Can you work these out from the model? Positions are in its coordinate system, mm. Face numbers are marked on the shaded views. A direction names the side the tool comes from. Give positions to 0.01 mm unless a question says otherwise; leave off trailing zeros. Loops run counter-clockwise (first coordinate to the right, second up) from the corner with the lowest first, then second, coordinate; pieces in that order, holes last. Notation, with made-up numbers: (20.5, -19.5) - (24.5, -19.5) arc R18 cw to (24.5, -0.5) - close; hole circle Ø9 at (55.25, 35.25). An arc over 180 degrees is marked (long way). Write item = value, one per line.
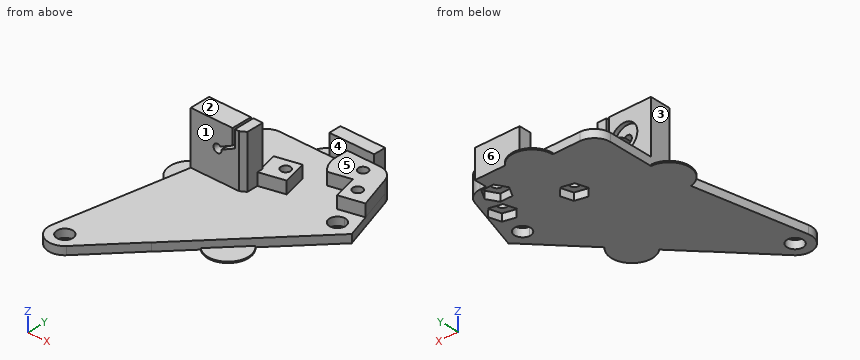
from build123d import *

# Parameters (mm, degrees)
SKETCH2_R                = 3.81
BOSS_EXTRUDE1_DEPTH      = 2.54
SKETCH5_W                = 16.764
SKETCH5_H                = 6.35
BOSS_EXTRUDE2_DEPTH      = 16.51
SKETCH6_R                = 4.1275
CUT_EXTRUDE2_DEPTH       = 1.27
SKETCH7_R                = 1.27
CUT_EXTRUDE3_DEPTH       = 65.77
CUT_EXTRUDE4_DEPTH       = 2.286
BOSS_EXTRUDE3_DEPTH      = 3.81
F_4_CLEARANCE_HOLE1_D    = 2.9464
SKETCH14_W               = 13.97
SKETCH14_H               = 3.81
BOSS_EXTRUDE6_DEPTH      = 6.35
BOSS_EXTRUDE6_DEPTH_BACK = 2.54
FILLET1_R                = 5.08
CUT_EXTRUDE5_DEPTH       = 17.51
CUT_EXTRUDE5_DEPTH_BACK  = 3.54
SKETCH19_R               = 2.4892
BOSS_EXTRUDE8_DEPTH      = 2.54
CUT_EXTRUDE8_DEPTH       = 2.54
CUT_EXTRUDE9_DEPTH       = 53.355501773
SKETCH13_R               = 6.35
PRINT_TABS_DEPTH         = 0.4


with BuildPart() as part:
    # Sketch2 → Boss-Extrude1 (new body)
    with BuildSketch(Plane.XY):
        with BuildLine():
            Line((-17.068825413, -8.459178389), (-41.402, 40.64))
            Line((-41.402, 40.64), (-41.402, 66.04))
            Line((-41.402, 66.04), (-1.524, 66.04))
            Line((-1.524, 66.04), (18.109053667, 5.913093546))
            ThreePointArc((18.109053667, 5.913093546), (7.204933647, -17.634949139), (-17.068825413, -8.459178389))
        make_face()
        Circle(SKETCH2_R, mode=Mode.SUBTRACT)
    extrude(amount=BOSS_EXTRUDE1_DEPTH)

    # Sketch5 → Boss-Extrude2 (add)
    with BuildSketch(Plane.XY.offset(2.54)):
        with Locations((-33.02, 43.815)):
            Rectangle(SKETCH5_W, SKETCH5_H)
    extrude(amount=BOSS_EXTRUDE2_DEPTH)

    # Sketch6 → Cut-Extrude2 (cut)
    with BuildSketch(Plane(origin=(0, 46.99, 0), x_dir=(1, 0, 0), z_dir=(0, 1, 0))):
        with Locations((-33.02, -11.43)):
            Circle(SKETCH6_R)
    extrude(amount=-CUT_EXTRUDE2_DEPTH, mode=Mode.SUBTRACT)

    # Sketch7 → Cut-Extrude3 (cut, through all)
    with BuildSketch(Plane(origin=(0, 45.72, 0), x_dir=(1, 0, 0), z_dir=(0, 1, 0))):
        with Locations((-33.02, -11.43)):
            Circle(SKETCH7_R)
    extrude(amount=-CUT_EXTRUDE3_DEPTH, mode=Mode.SUBTRACT)

    # Sketch9 → Cut-Extrude4 (cut)
    with BuildSketch(Plane(origin=(0, 0, 0), x_dir=(-1, 0, 0), z_dir=(0, 0, -1))):
        Polygon((3.171122265, 62.23), (5.077532854, 58.928), (8.890354032, 58.928), (10.796764621, 62.23), (8.890354032, 65.532), (5.077532854, 65.532), align=None)
        Polygon((24.379877895, 49.663956202), (23.308143816, 53.323053276), (19.603405755, 54.224452874), (16.970401774, 51.466755398), (18.042135853, 47.807658324), (21.746873914, 46.906258726), align=None)
        Polygon((5.918476139, 54.15579827), (4.846742059, 57.814895344), (1.142003999, 58.716294942), (-1.490999983, 55.958597466), (-0.419265903, 52.299500392), (3.285472157, 51.398100794), align=None)
    extrude(amount=-CUT_EXTRUDE4_DEPTH, mode=Mode.SUBTRACT)

    # Sketch8 → Boss-Extrude3 (add)
    with BuildSketch(Plane.XY.offset(2.54)):
        with BuildLine():
            Line((-15.367, 66.04), (-6.983943443, 66.04))
            Line((-6.983943443, 66.04), (-1.524, 66.04))
            Line((-1.524, 66.04), (3.09175139, 51.904101595))
            Line((3.09175139, 51.904101595), (-4.240438106, 50.120107003))
            Line((-4.240438106, 50.120107003), (-6.088713216, 57.716488409))
            Line((-6.088713216, 57.716488409), (-12.708473154, 56.10583501))
            ThreePointArc((-12.708473154, 56.10583501), (-14.673699407, 58.891843255), (-15.367, 62.23))
            Line((-15.367, 62.23), (-15.367, 66.04))
        make_face()
        Polygon((-17.142042414, 46.981018422), (-18.990317524, 54.577399829), (-26.415687706, 52.770733449), (-24.567412596, 45.174352043), align=None)
    extrude(amount=BOSS_EXTRUDE3_DEPTH)

    # #4 Clearance Hole1 (through all)
    with Locations(Plane.XY.offset(6.35)):
        with Locations((-6.983943443, 62.23), (-20.675139834, 50.5653558), (-2.213738078, 55.057197868)):
            Hole(F_4_CLEARANCE_HOLE1_D / 2)

    # Sketch14 → Boss-Extrude6 (add, two sides)
    with BuildSketch(Plane.XY.offset(2.54)) as boss_extrude6_sk:
        with Locations((-13.968943443, 67.945)):
            Rectangle(SKETCH14_W, SKETCH14_H)
    extrude(amount=BOSS_EXTRUDE6_DEPTH)
    extrude(boss_extrude6_sk.sketch, amount=-BOSS_EXTRUDE6_DEPTH_BACK)

    # Fillet1
    fillet1_edges = [part.edges().sort_by_distance(p)[0] for p in [
        (-1.524, 66.04, 3.175),
        (-41.402, 66.04, 1.27),
    ]]
    fillet(fillet1_edges, radius=FILLET1_R)

    # Sketch15 → Cut-Extrude5 (cut, two sides)
    with BuildSketch(Plane.XY.offset(2.54)) as cut_extrude5_sk:
        with BuildLine():
            ThreePointArc((-0.315167053, 48.411374113), (-18.310138041, 44.816284079), (-33.674369734, 34.782140486))
            ThreePointArc((-33.674369734, 34.782140486), (-33.731327517, 31.262340905), (-30.211527936, 31.205383122))
            ThreePointArc((-30.211527936, 31.205383122), (-16.427248714, 40.207684038), (-0.28275743, 43.433079608))
            ThreePointArc((-0.28275743, 43.433079608), (2.190185011, 45.938431672), (-0.315167053, 48.411374113))
        make_face()
    extrude(amount=CUT_EXTRUDE5_DEPTH, mode=Mode.SUBTRACT)
    extrude(cut_extrude5_sk.sketch, amount=-CUT_EXTRUDE5_DEPTH_BACK, mode=Mode.SUBTRACT)

    # Sketch19 → Boss-Extrude8 (add, through all)
    with BuildSketch(Plane.XY.offset(2.54)):
        with BuildLine():
            Line((5.466200245, 44.632269783), (-40.158007355, -3.769954845))
            ThreePointArc((-40.158007355, -3.769954845), (-46.15516131, -4.814733016), (-48.848797168, 0.64436424))
            Line((-48.848797168, 0.64436424), (-41.402, 40.64))
            Line((-41.402, 40.64), (3.09175139, 51.904101595))
            Line((3.09175139, 51.904101595), (5.466200245, 44.632269783))
        make_face()
        with Locations((-0.298962241, 45.92222686)):
            Circle(SKETCH19_R, mode=Mode.SUBTRACT)
        with Locations((-43.854625645, -0.285501773)):
            Circle(SKETCH19_R, mode=Mode.SUBTRACT)
    extrude(amount=-BOSS_EXTRUDE8_DEPTH)

    # Sketch20 → Cut-Extrude8 (cut)
    with BuildSketch(Plane.XY.offset(2.54)):
        Polygon((-40.158007355, -3.769954845), (10.729493517, 49.863783044), (48.07174347, 14.433588323), (-7.673080914, -44.319607422), align=None)
    extrude(amount=-CUT_EXTRUDE8_DEPTH, mode=Mode.SUBTRACT)

    # Sketch21 → Cut-Extrude9 (cut, through all)
    with BuildSketch(Plane(origin=(0, 46.99, 0), x_dir=(1, 0, 0), z_dir=(0, 1, 0))):
        Polygon((-27.559, -19.05), (-27.559, -13.73452905), (-32.84961162, -11.08922324), (-33.19038838, -11.77077676), (-28.321, -14.20547095), (-28.321, -19.05), align=None)
    extrude(amount=-CUT_EXTRUDE9_DEPTH, mode=Mode.SUBTRACT)

    # Sketch13 → Print Tabs (add)
    with BuildSketch(Plane(origin=(0, 0, 0), x_dir=(-1, 0, 0), z_dir=(0, 0, -1))):
        with Locations((14.284313144, 23.500060577)):
            Circle(SKETCH13_R)
        with Locations((21.463, 66.04)):
            Circle(SKETCH13_R)
        with Locations((41.402, 40.64)):
            Circle(SKETCH13_R)
    extrude(amount=-PRINT_TABS_DEPTH)


solid = part.part
Q1. We'd pull the mould along Y, two halves only. Please class the marked faces 4, 5 and 6: released by +Y, released by -Y, zero draft, split by the parting line, or undercut.
Output:
face_4 = undercut
face_5 = zero draft
face_6 = released by +Y
Q2. Imagine slicing it at B-B, the plane z = 18. Write out the boundary of the cut face in (x, y), then the cut area to 3 significant figures.
Output:
outline = (-41.4, 40.64) - (-28.32, 40.64) - (-28.32, 46.99) - (-41.4, 46.99) - close; (-27.56, 40.64) - (-26.31, 40.64) arc R48.41 cw to (-24.64, 41.67) - (-24.64, 46.99) - (-27.56, 46.99) - close
area = 101 mm2
Q3. Imagine slicing it at D-D, the plane x = -2. Write out the boundary of the cut face in (y, z), then the cut area to 3 significant figures.
Output:
outline = (36.45, 0) - (44.1, 0) - (44.1, 2.54) - (36.45, 2.54) - close; (47.74, 0) - (51.71, 0) - (51.71, 2.29) - (53.6, 2.29) - (53.6, 6.35) - (50.67, 6.35) - (50.67, 2.54) - (47.74, 2.54) - close; (56.51, 2.29) - (58.51, 2.29) - (58.51, 0) - (64.9, 0) - (64.9, 6.35) - (56.51, 6.35) - close
area = 89.9 mm2
Q4. For pin 1 (4 mm diameter, centred on y = 63, z = 4, fed in from -X); pin 2 (7.5 mm diameter, centred on x = -33.02, z = 11.43, fed in from +Y); pin 3 (1.9 mm diameter, centred on x = -14.5, z = 6.5, fed in from -Y); pin 4 (6 mm diameter, centred on y = 37, z = 15.5, fed in from +X), each with a flat end and sliding along its axis, tell me the tip position at first contact or that it passes through.
Output:
pin_1 = -41.36
pin_2 = 45.72
pin_3 = 57.03
pin_4 = through
Q5. Imagine slicing it at C-C, the plane z = 4.75. Write out the boundary of the cut face in (x, y), then the cut area to 3 significant figures.
Output:
outline = (-41.4, 40.64) - (-26.31, 40.64) arc R48.41 cw to (-24.64, 41.67) - (-24.64, 45.46) - (-24.57, 45.17) - (-17.14, 46.98) - (-18.99, 54.58) - (-26.42, 52.77) - (-25.01, 46.99) - (-41.4, 46.99) - close; (-20.95, 66.04) - (-15.37, 66.04) - (-15.37, 62.23) arc R8.38 ccw to (-12.71, 56.11) - (-6.09, 57.72) - (-4.24, 50.12) - (3.09, 51.9) - (-0.38, 62.54) arc R5.08 ccw to (-5.21, 66.04) - (-6.98, 66.04) - (-6.98, 69.85) - (-20.95, 69.85) - close; hole circle Ø2.95 at (-20.68, 50.57); hole circle Ø2.95 at (-6.98, 62.23); hole circle Ø2.95 at (-2.21, 55.06)
area = 377 mm2
Q6. I need wall thicknesses on L1, parallel to X at y = 44.3, z = 11.43; L2, parallel to Z at x = -33.02, y = 43.3; L3, parallel to Z at x = -33.5, y = 60. Which ranges of each line are inside material? Lowest first, please.
Output:
L1 = -41.4 to -34.29, -31.75 to -24.64
L2 = 0 to 10.16, 12.7 to 19.05
L3 = 0 to 2.54
Q7. Which directions (+Z, -Z, +X, -X, +Y, -Y) give clear straight access to the entire face, cutting with the end or side of a thin tool? Please do the marked faces 1, 2 and 3.
Output:
face_1 = +Z, +X, -X, -Y
face_2 = +Z, +X, -X, +Y, -Y
face_3 = +Z, -X, +Y
Q8. Imagine slicing it at A-A, the plane x = -33.02. Write out the boundary of the cut face in (y, z).
Output:
outline = (3.8, 0) - (66.04, 0) - (66.04, 2.54) - (46.99, 2.54) - (46.99, 7.3) - (45.72, 7.3) - (45.72, 10.16) - (40.64, 10.16) - (40.64, 2.54) - (3.8, 2.54) - close; (40.64, 12.7) - (45.72, 12.7) - (45.72, 15.56) - (46.99, 15.56) - (46.99, 19.05) - (40.64, 19.05) - close
